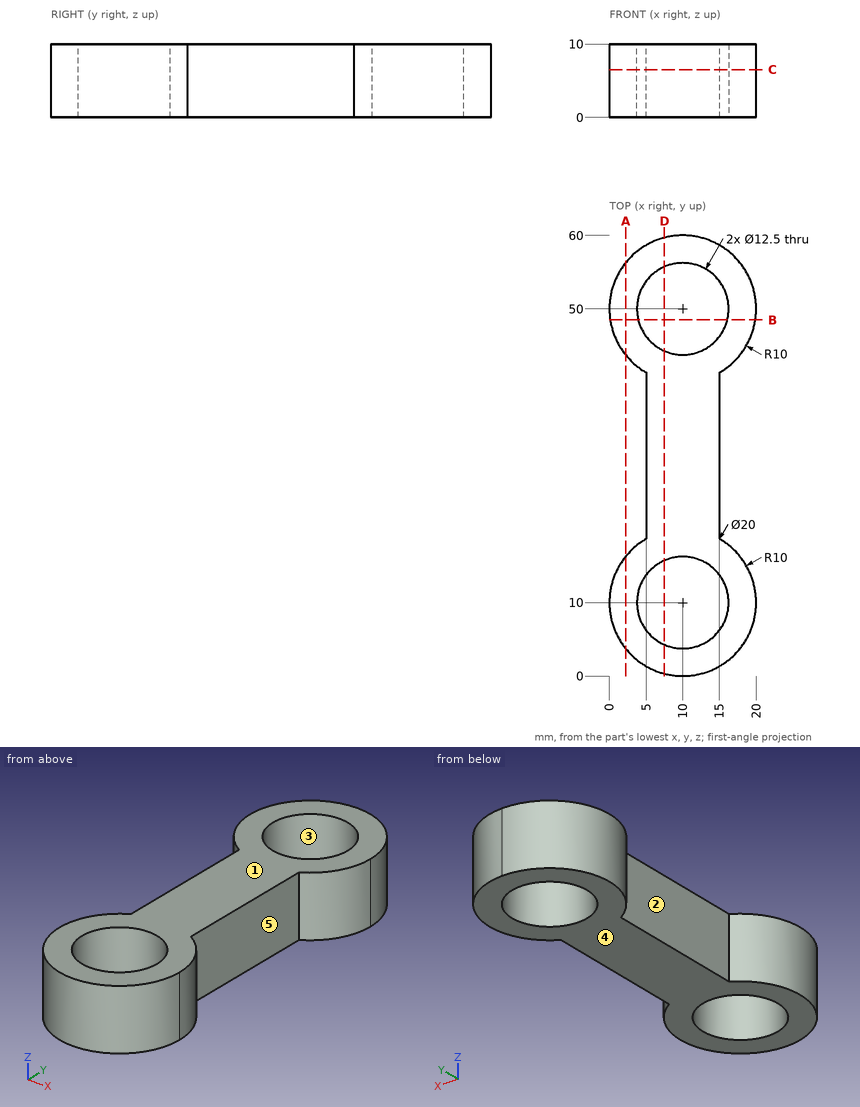
Study the drawing (mm; zero at the part's minimum x, y, z) and answer. A direction names the side the tool comes from. Coordinates: 2 decimals unless noted, no trailing zeros. Write each loop counter-clockwise with the first axis right and the second up, starting at its lowest first coordinate (ties: lowest second). Pieces come first, ordered by that corner, then holes. Notation, with made-up numbers: (-36.5, -15) -> (-11.5, -15) arc R14 ccw to (-11.5, 3) -> close; hole circle Ø8 at (-20.75, 48.25). An arc over 180 degrees is marked (long way). Write each question's results on one line, items separated by ' | '. Start each with the question number.
1) A cutting plane is placed at D-D (x = 7.5). Determine the outline of the cut face in (y, z).
2) Flat-ended cylindrical pins translate along their axes: pin 1 Ø5 at (y, z) = (35.5, 6) entering from +X; pin 2 Ø3 at (y, z) = (30.5, 6) entering from -X; pin 3 Ø1.5 at (x, z) = (8.5, 1.5) entering from -Y; pin 4 Ø6 at (x, y) = (6.5, 50) entering from +Z. Find the tip coordinate at first contact, or state that the pin passes through.
3) Straight lines are drawn through the part: probe 1 along Y at (x, z) = (11.5, 2.5); probe 2 along Y at (x, z) = (6.5, 7); probe 3 along X at (y, z) = (30, 9.75). For each, find the intervals that lie inside material, in ascending order.
4) A cutting plane is placed at A-A (x = 2.25). Determine the outline of the cut face in (y, z), then the cut area to 3 significant figures.
5) A cutting plane is placed at C-C (z = 6.5). Determine the outline of the cut face in (x, y).
6) A tool of negligible diameter and unlimited length cuts with its end or side. For the marked faces 4 and 5, from which of +Z, -Z, +X, -X, +Y, -Y can it reach the whole face along a straight path? Write none if from no direction.
7) A cutting plane is placed at B-B (y = 48.5). Determine the outline of the cut face in (x, z).
8) For a pull along Y with two mould halves and no side action, classify the marked faces 1, 2 and 3 as +Y half, -Y half, draft (parallel to the pull), parting line (faces both ways), or undercut.
Values follow:
1) outline: (0.32, 0) -> (4.27, 0) -> (4.27, 10) -> (0.32, 10) -> close; (15.73, 0) -> (44.27, 0) -> (44.27, 10) -> (15.73, 10) -> close; (55.73, 0) -> (59.68, 0) -> (59.68, 10) -> (55.73, 10) -> close
2) pin 1: x = 15 | pin 2: x = 5 | pin 3: y = 0.03 | pin 4: z = 10
3) probe 1: 0.11 to 3.93, 16.07 to 43.93, 56.07 to 59.89 | probe 2: 0.63 to 4.82, 15.18 to 44.82, 55.18 to 59.37 | probe 3: 5 to 15
4) outline: (3.68, 0) -> (16.32, 0) -> (16.32, 10) -> (3.68, 10) -> close; (43.68, 0) -> (56.32, 0) -> (56.32, 10) -> (43.68, 10) -> close | area: 253 mm²
5) outline: (5, 18.66) arc R10 ccw (long way) to (15, 18.66) -> (15, 41.34) arc R10 ccw (long way) to (5, 41.34) -> close; hole circle Ø12.5 at (10, 10); hole circle Ø12.5 at (10, 50)
6) face 4: -Z, +X, -X, +Y, -Y | face 5: +Z, -Z, +X
7) outline: (0.11, 0) -> (3.93, 0) -> (3.93, 10) -> (0.11, 10) -> close; (16.07, 0) -> (19.89, 0) -> (19.89, 10) -> (16.07, 10) -> close
8) face 1: draft | face 2: undercut | face 3: undercut
